Here's how the part is built. I have some questions about the finished solid (model axes, mm). A direction names the side the tool comes from. Round coordinates to 2 decimals unless told otherwise and drop trailing zeros. Write each loop counter-clockwise with the first axis right and the second up, starting at its lowest first coordinate (ties: lowest second). Pieces come first, ordered by that corner, then holes. Notation, with made-up numbers: (-16, -16) -> (23, -16) arc R15 ccw to (23, -4) -> close; hole circle Ø7 at (-1, 32.25). An arc over 180 degrees is marked (long way). Answer as CSV lines item,"result".
from build123d import *

# Parameters (mm, degrees)
F0_W      = 30
F0_H      = 30
F1_DEPTH  = 15
F2_W      = 90
F2_H      = 90
F3_DEPTH  = 3
F4_R      = 5
F5_DEPTH  = 3.001
F6_R      = 3
F7_DEPTH  = 5
F8_SIZE   = 1
F9_R      = 3.05
F10_DEPTH = 5.2


with BuildPart() as f1:
    # F0 (on Top) → F1 (new body)
    with BuildSketch(Plane.XY):
        Rectangle(F0_W, F0_H)
    extrude(amount=F1_DEPTH)

    # F2 (on Top) → F3 (join)
    with BuildSketch(Plane.XY):
        Rectangle(F2_W, F2_H)
    extrude(amount=-F3_DEPTH)

    # F4 (on face) → F5 (cut, through all)
    with BuildSketch(Plane.XY):
        with Locations((-36, 36)):
            Circle(F4_R)
        with Locations((36, 36)):
            Circle(F4_R)
        with Locations((36, -36)):
            Circle(F4_R)
        with Locations((-36, -36)):
            Circle(F4_R)
    extrude(amount=-F5_DEPTH, mode=Mode.SUBTRACT)

    # F6 (on face) → F7 (join)
    with BuildSketch(Plane.XY.offset(15)):
        with Locations((-6, 6)):
            Circle(F6_R)
        with Locations((6, -6)):
            Circle(F6_R)
    extrude(amount=F7_DEPTH)

    # F8
    f8_edges = [f1.edges().sort_by_distance(p)[0] for p in [
        (-9, 6, 20),
        (3, -6, 20),
    ]]
    chamfer(f8_edges, length=F8_SIZE)

    # F9 (on face) → F10 (cut)
    with BuildSketch(Plane.XY.offset(15)):
        with Locations((-6, -6)):
            Circle(F9_R)
        with Locations((6, 6)):
            Circle(F9_R)
    extrude(amount=-F10_DEPTH, mode=Mode.SUBTRACT)


solid = f1.part
Item 1: Suppose I cut it at D-D, the plane y = -6. List the corners of the cut face in (x, z) for me, then the cut area to 3 significant figures.
Results found:
outline,"(-45, -3) -> (45, -3) -> (45, 0) -> (15, 0) -> (15, 15) -> (9, 15) -> (9, 19) -> (8, 20) -> (4, 20) -> (3, 19) -> (3, 15) -> (-2.95, 15) -> (-2.95, 9.8) -> (-9.05, 9.8) -> (-9.05, 15) -> (-15, 15) -> (-15, 0) -> (-45, 0) -> close"
area,"717 mm²"
Item 2: Suppose I cut it at A-A, the plane x = -36. List the corners of the cut face in (y, z) for me, then the cut area to 3 significant figures.
Results found:
outline,"(-45, -3) -> (-41, -3) -> (-41, 0) -> (-45, 0) -> close; (-31, -3) -> (31, -3) -> (31, 0) -> (-31, 0) -> close; (41, -3) -> (45, -3) -> (45, 0) -> (41, 0) -> close"
area,"210 mm²"
Item 3: If we mould it in two halves opening along Y, with no side actions, what happens to faces 4 (the cylindrical face through (-4.593, -8.706, 12.436)), 5 (the flat face through (-6, -6, 9.8)), 6 (the flat face through (-1, 45, -1)), 7 (the flat face through (-6, 6, 20))? For each: pulls with the +Y half, pulls with the -Y half, needs draft (parallel to the pull), parting line crosses it, or undercut.
Results found:
face 4,"undercut"
face 5,"undercut"
face 6,"pulls with the +Y half"
face 7,"needs draft"
Item 4: Suppose I cut it at C-C, the plane z = -1.5. List the corners of the cut face in (x, y) for me.
Results found:
outline,"(-45, -45) -> (45, -45) -> (45, 45) -> (-45, 45) -> close; hole circle Ø10 at (-36, -36); hole circle Ø10 at (-36, 36); hole circle Ø10 at (36, -36); hole circle Ø10 at (36, 36)"
Item 5: I need wall thicknesses on L1, parallel to Y at x = 36, z = -2; L2, parallel to Y at x = 6, z = 12.2; L3, parallel to Y at x = -6, z = 12. Which ranges of each line are inside material? Lowest first, please.
Results found:
L1,"y = -45 to -41, -31 to 31, 41 to 45"
L2,"y = -15 to 2.95, 9.05 to 15"
L3,"y = -15 to -9.05, -2.95 to 15"
Item 6: Will these pins go through, and if not, where does the flat tip stop? pin 1 (6 mm diameter, centred on x = -6, y = -20.5, fed in from +Z); pin 2 (6.5 mm diameter, centred on x = 5.5, y = 6.5, fed in from +Z); pin 3 (5.5 mm diameter, centred on x = 6, y = 6, fed in from +Z).
Results found:
pin 1,"stops at z = 0"
pin 2,"stops at z = 15"
pin 3,"stops at z = 9.8"
Item 7: For faces 1 (the flat face through (-15, 0, 7)), 2 (the cylindrical face through (5.339, 3.023, 12.436)), 3 (the cylindrical face through (-41, -36, -1)), which set-ups out of +Z, -Z, +X, -X, +Y, -Y let a thin tool reach every point of the face, with its end or its side?
Results found:
face 1,"+Z, -X, +Y, -Y"
face 2,"+Z"
face 3,"+Z, -Z"
